Print and shaded views of the part. All mm, measured from the part's lowest x, y and z. Coordinates: 2 decimals unless noted, no trailing zeros. Order: outer loops, then holes, each group sorted by start corner. A loop starts at its lowest first (then second) coordinate and runs counter-clockwise, first axis right, second up. Notation, with made-up numbers: (7, 9) -> (35, 9) arc R26 cw to (35, 29) -> close; hole circle Ø11 at (71.25, -22). An arc over 180 degrees is marked (long way). Return JSON: item names as keys, results as strings. Group by question number.
1) Probe line 1 (X direction, y = 1.9, z = 27); line 2 (Z direction, x = 10.25, y = 4.4); line 3 (X direction, y = 1.95, z = 21). List the from-to ranges inside material, lowest first.
2) Cut at C-C (y = 1.8). Write the cut outline in (x, z).
3) Cut at A-A (z = 27). Write the cut outline in (x, y).
4) Cut at B-B (x = 15). Write the cut outline in (y, z), and give its area (3 significant figures).
5) Pull direction X, two halves, no side cores. Call the marked faces 1, 2 and 3: +X half, -X half, draft (parallel to the pull), parting line (faces both ways), or undercut.
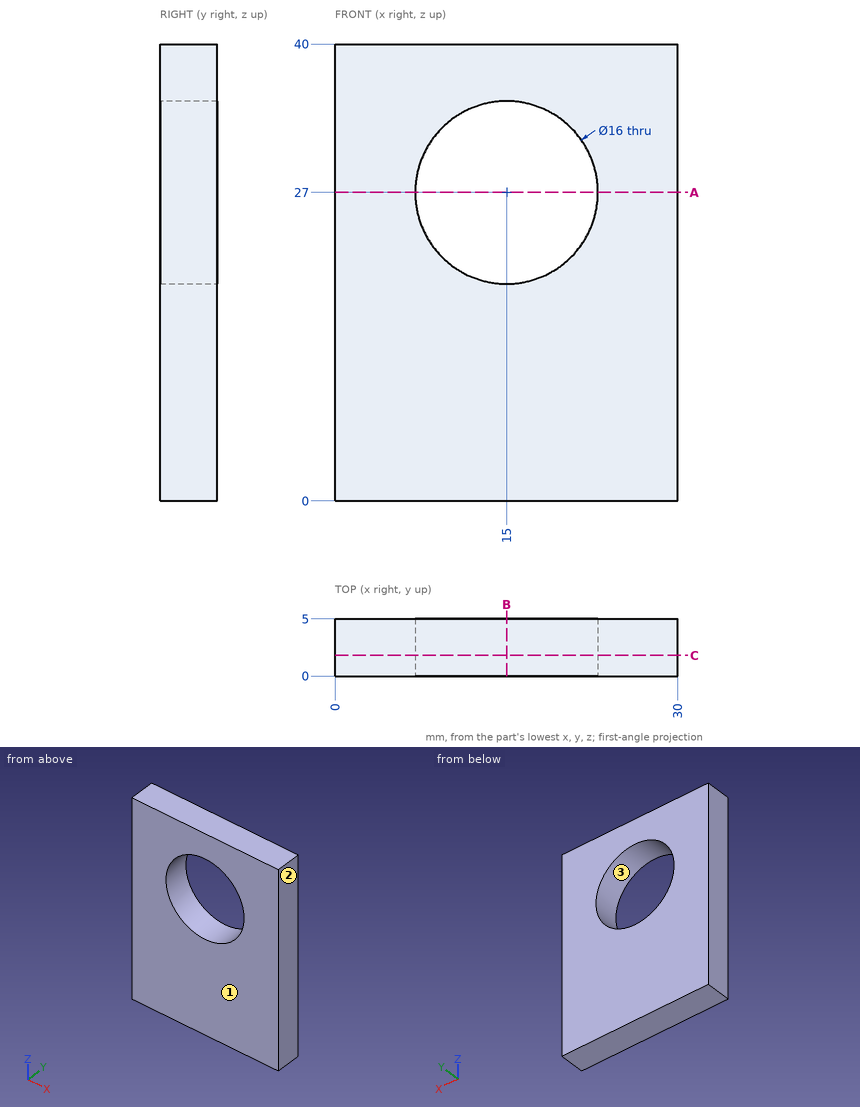
Answers below:
{
 "1": {"line 1": "x = 0 to 7, 23 to 30", "line 2": "z = 0 to 20.56, 33.44 to 40", "line 3": "x = 0 to 9.71, 20.29 to 30"},
 "2": {"outline": "(0, 0) -> (30, 0) -> (30, 40) -> (0, 40) -> close; hole circle Ø16 at (15, 27)"},
 "3": {"outline": "(0, 0) -> (7, 0) -> (7, 5) -> (0, 5) -> close; (23, 0) -> (30, 0) -> (30, 5) -> (23, 5) -> close"},
 "4": {"outline": "(0, 0) -> (5, 0) -> (5, 19) -> (0, 19) -> close; (0, 35) -> (5, 35) -> (5, 40) -> (0, 40) -> close", "area": "120 mm^2"},
 "5": {"face 1": "draft", "face 2": "+X half", "face 3": "undercut"}
}
